Read the model definition and answer for the solid it produces. Units are mm, in the model's axes. A direction names the side the tool comes from. Coordinates: 2 decimals unless noted, no trailing zeros. Write each loop counter-clockwise with the first axis right and the second up, starting at its lowest first coordinate (ties: lowest second). Pieces come first, ordered by that corner, then holes.
Item 1: Each of these flat-tipped pins is pushed along its axis until it touches: P1, Ø1.9, axis at y = -4.5, z = 10, coming from the +X side; P2, Ø1.9, axis at x = -27, y = 0, coming from the +Z side; P3, Ø1.5, axis at y = -1.5, z = -5.5, coming from the -X side. Where does it stop, or does it pass through?
Item 2: Determine the mould class of faces 1 (the face through (28.514, -2.888, -0.336)), 2 (the face through (-30, 0.1, 24.5)), 3 (the face through (-30.5, 0.1, -0.4)), 4 (the face through (-0.1, -6.2, -25)) for opening direction Y: released by +Y, released by -Y, zero draft, split by the parting line, or undercut.
Item 3: A tool of negligible diameter and unlimited length cuts with its end or side. For faces 5 (the face through (2.1, -5.7, -24)), 6 (the face through (0, -6.5, 0)), 7 (the face through (25, -5.41, -0.34)), from which of +Z, -Z, +X, -X, +Y, -Y can it reach the whole face along a straight path? Write none if from no direction.
Item 4: Section A-A (x = -12) is taken. Give the vertices of the cut face in (y, z).
Item 5: Straight lines are drawn through the part: probe 1 along X at (y, z) = (0, -4); probe 2 along Y at (x, z) = (8.5, -1); probe 3 along Y at (x, z) = (-27, -13). For each, find the intervals that lie inside material, in ascending order.
Item 6: Section C-C (y = 3.75) is taken. Give the vertices of the cut face in (x, z), then the cut area to 3 significant figures.
from build123d import *

# Parameters (mm, degrees)
BOSS_EXTRUDE1_DEPTH      = 25
BOSS_EXTRUDE1_DEPTH_BACK = 25
CUT_EXTRUDE1_DEPTH       = 1


with BuildPart() as part:
    # Sketch1 → Boss-Extrude1 (new, two sides: drawn at the far end of the back side and taken through both)
    with BuildSketch(Plane.XY.offset(-BOSS_EXTRUDE1_DEPTH_BACK)):
        with BuildLine():
            Line((24, 6.5), (-24, 6.5))
            ThreePointArc((-24, 6.5), (-30.5, 0), (-24, -6.5))
            Line((-24, -6.5), (24, -6.5))
            ThreePointArc((24, -6.5), (30.5, 0), (24, 6.5))
        make_face()
        with BuildLine():
            Line((24, 5.5), (-24, 5.5))
            ThreePointArc((-24, 5.5), (-26.564388223, 4.865584553), (-28.537180991, 3.108695652))
            ThreePointArc((-28.537180991, 3.108695652), (-28.590919755, 2.180372836), (-27.794733192, 1.7))
            Line((-27.794733192, 1.7), (-27, 1.7))
            ThreePointArc((-27, 1.7), (-26.292893219, 1.407106781), (-26, 0.7))
            Line((-26, 0.7), (-26, 0.5))
            Line((-26, 0.5), (-26.440983006, 0.5))
            ThreePointArc((-26.440983006, 0.5), (-27.75, 0), (-26.440983006, -0.5))
            Line((-26.440983006, -0.5), (-26, -0.5))
            Line((-26, -0.5), (-26, -2.325))
            Line((-26, -2.325), (-26.555673326, -2.325))
            ThreePointArc((-26.555673326, -2.325), (-28.515, -2.85), (-26.555673326, -3.375))
            Line((-26.555673326, -3.375), (-26, -3.375))
            Line((-26, -3.375), (-26, -5.123475383))
            ThreePointArc((-26, -5.123475383), (-25.017567048, -5.405049242), (-24, -5.5))
            Line((-24, -5.5), (24, -5.5))
            ThreePointArc((24, -5.5), (25.017567048, -5.405049242), (26, -5.123475383))
            Line((26, -5.123475383), (26, -3.375))
            Line((26, -3.375), (26.555673326, -3.375))
            ThreePointArc((26.555673326, -3.375), (28.515, -2.85), (26.555673326, -2.325))
            Line((26.555673326, -2.325), (26, -2.325))
            Line((26, -2.325), (26, -0.5))
            Line((26, -0.5), (26.440983006, -0.5))
            ThreePointArc((26.440983006, -0.5), (27.75, 0), (26.440983006, 0.5))
            Line((26.440983006, 0.5), (26, 0.5))
            Line((26, 0.5), (26, 0.7))
            ThreePointArc((26, 0.7), (26.292893219, 1.407106781), (27, 1.7))
            Line((27, 1.7), (27.794733192, 1.7))
            ThreePointArc((27.794733192, 1.7), (28.590919755, 2.180372836), (28.537180991, 3.108695652))
            ThreePointArc((28.537180991, 3.108695652), (26.564388223, 4.865584553), (24, 5.5))
        make_face(mode=Mode.SUBTRACT)
    extrude(amount=BOSS_EXTRUDE1_DEPTH + BOSS_EXTRUDE1_DEPTH_BACK)

    # Sketch2 → Cut-Extrude1 (cut)
    with BuildSketch(Plane.XY.offset(25)):
        with BuildLine():
            Line((24, 6), (-24, 6))
            ThreePointArc((-24, 6), (-30, 0), (-24, -6))
            Line((-24, -6), (24, -6))
            ThreePointArc((24, -6), (30, 0), (24, 6))
        make_face()
    cut_extrude1 = extrude(amount=-CUT_EXTRUDE1_DEPTH, mode=Mode.SUBTRACT)

    # Mirror1: Cut-Extrude1 across plane
    add(cut_extrude1.mirror(Plane.XY), mode=Mode.SUBTRACT)


solid = part.part
Established:
1. P1: stops at x = 29.44
1. P2: stops at z = 24
1. P3: stops at x = -30.46
2. face 1: undercut
2. face 2: undercut
2. face 3: split by the parting line
2. face 4: zero draft
3. face 5: -Z
3. face 6: +Z, -Z, +X, -X, -Y
3. face 7: +Z, -Z
4. outline: (-6.5, -25) - (-6, -25) - (-6, -24) - (-5.5, -24) - (-5.5, 24) - (-6, 24) - (-6, 25) - (-6.5, 25) - close; (5.5, -24) - (6, -24) - (6, -25) - (6.5, -25) - (6.5, 25) - (6, 25) - (6, 24) - (5.5, 24) - close
5. probe 1: x = -30.5 to -27.75, 27.75 to 30.5
5. probe 2: y = -6.5 to -5.5, 5.5 to 6.5
5. probe 3: y = -5.77 to -3.79, -1.91 to -0.75, 0.75 to 1.7, 4.61 to 5.77
6. outline: (-29.31, -25) - (-28.68, -25) - (-28.68, -24) - (-28.02, -24) - (-28.02, 24) - (-28.68, 24) - (-28.68, 25) - (-29.31, 25) - close; (28.02, -24) - (28.68, -24) - (28.68, -25) - (29.31, -25) - (29.31, 25) - (28.68, 25) - (28.68, 24) - (28.02, 24) - close
6. area: 126 mm2
